Geometry: final body of the model. Coordinates: model frame, mm. A direction names the side the tool comes from. Coordinates: 2 decimals unless noted, no trailing zeros. Write item = value, one per line. Start each with the question number.
Item 1: Reachability of faces 1 (the flat face through (0, 0, 3)), 2 (the flat face through (263.4, 6, 3)) from +Z, -Z, +X, -X, +Y, -Y: full face, straight path, thin tool, end or side. Return the list, or none.
Item 2: Pull-direction query (Y, two-part tool) for faces 3 (the flat face through (267.6, 6, 3)), 4 (the flat face through (135, 1, 0)), 5 (the flat face through (135, -43.7, 3)); classes: +Y half, -Y half, draft (parallel to the pull), parting line (faces both ways), or undercut.
Item 3: Ray query, L1, parallel to Y at x = 17, z = 4.2; L2, parallel to X at y = 5.5, z = 5; L3, parallel to X at y = 38.5, z = 3.4. Return the intervals inside material, ascending. Write a range as [from, to].
Item 4: First-contact query: pin 1 Ø5 at (x, y) = (265.5, 16.45) entering from -Z; pin 2 Ø2 at (x, z) = (266, 2) entering from -Y. Flat tips, straight axial feed; report the tip coordinate or a pass-through.
from build123d import *

# Parameters (mm, degrees)
BOSS_EXTRUDE1_DEPTH = 5.8
SKETCH3_W           = 4.2
SKETCH3_H           = 12
CUT_EXTRUDE1_DEPTH  = 6.35
SKETCH4_R           = 1.55
CUT_EXTRUDE2_DEPTH  = 6.8
SKETCH5_R           = 1.55
CUT_EXTRUDE3_DEPTH  = 6.8


with BuildPart() as part:
    # Sketch2 → Boss-Extrude1 (new body)
    with BuildSketch(Plane.XY):
        with BuildLine():
            Line((263, 43.7), (10, 43.7))
            ThreePointArc((10, 43.7), (2.928932188, 40.771067812), (0, 33.7))
            Line((0, 33.7), (0, -33.7))
            ThreePointArc((0, -33.7), (2.928932188, -40.771067812), (10, -43.7))
            Line((10, -43.7), (263, -43.7))
            ThreePointArc((263, -43.7), (270.071067812, -40.771067812), (273, -33.7))
            Line((273, -33.7), (273, 33.7))
            ThreePointArc((273, 33.7), (270.071067812, 40.771067812), (263, 43.7))
        make_face()
    extrude(amount=BOSS_EXTRUDE1_DEPTH)

    # Sketch3 → Cut-Extrude1 (cut)
    with BuildSketch(Plane.XY.offset(5.8)):
        with Locations((265.5, 6)):
            Rectangle(SKETCH3_W, SKETCH3_H)
    extrude(amount=-CUT_EXTRUDE1_DEPTH, mode=Mode.SUBTRACT)

    # Sketch4 → Cut-Extrude2 (cut, through all)
    with BuildSketch(Plane.XY.offset(5.8)):
        with Locations((17, 32.5)):
            Circle(SKETCH4_R)
        with Locations((17, 18.5)):
            Circle(SKETCH4_R)
        with Locations((17, -18.5)):
            Circle(SKETCH4_R)
        with Locations((17, -32.5)):
            Circle(SKETCH4_R)
    extrude(amount=-CUT_EXTRUDE2_DEPTH, mode=Mode.SUBTRACT)

    # Sketch5 → Cut-Extrude3 (cut, through all)
    with BuildSketch(Plane.XY.offset(5.8)):
        with Locations((265.5, 16.45)):
            Circle(SKETCH5_R)
        with Locations((265.5, -9.55)):
            Circle(SKETCH5_R)
    extrude(amount=-CUT_EXTRUDE3_DEPTH, mode=Mode.SUBTRACT)


solid = part.part
Responses:
q1.face_1 = +Z, -Z, -X, +Y, -Y
q1.face_2 = +Z, -Z
q2.face_3 = undercut
q2.face_4 = draft
q2.face_5 = -Y half
q3.L1 = [-43.7, -34.05], [-30.95, -20.05], [-16.95, 16.95], [20.05, 30.95], [34.05, 43.7]
q3.L2 = [0, 263.4], [267.6, 273]
q3.L3 = [1.23, 271.77]
q4.pin_1 = 0
q4.pin_2 = -43.5
